The listing builds one solid part. Answer for the finished solid, in the listing's coordinates (mm). Face numbers are marked on the shaded views. A direction names the side the tool comes from. Give positions to 0.01 mm unless a question says otherwise; leave off trailing zeros. Write each loop counter-clockwise with the first axis right and the second up, starting at its lowest first coordinate (ties: lowest second). Pieces come first, ordered by that corner, then holes. Notation, with made-up numbers: (46.5, 62) - (102.5, 62) arc R17 cw to (102.5, 71) - close; hole circle Ø7 at (-27.5, 65.5). An arc over 180 degrees is marked (long way). Return JSON: item names as keys, results as strings.
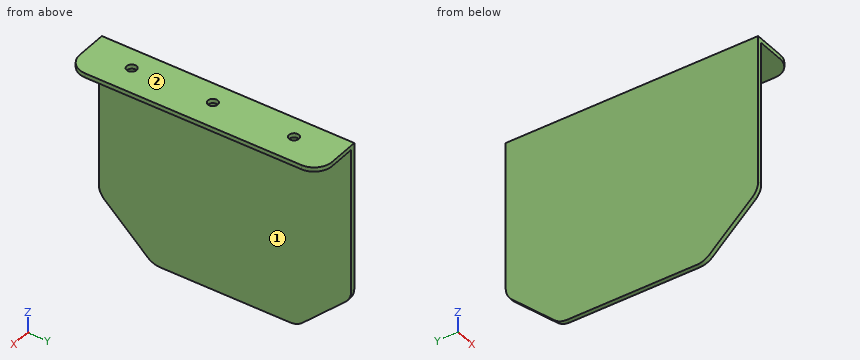
from build123d import *

# Parameters (mm, degrees)
SKETCH1_W           = 115
SKETCH1_H           = 140
BOSS_EXTRUDE1_DEPTH = 2.4
CUT_EXTRUDE1_DEPTH  = 3.4
FILLET1_R           = 10
SKETCH3_W           = 2.4
SKETCH3_H           = 140
BOSS_EXTRUDE2_DEPTH = 25
FILLET2_R           = 10
SKETCH4_R           = 2.75
CUT_EXTRUDE2_DEPTH  = 116


with BuildPart() as part:
    # Sketch1 → Boss-Extrude1 (new body)
    with BuildSketch(Plane(origin=(0, 0, 0), x_dir=(0, 0, -1), z_dir=(1, 0, 0))):
        with Locations((57.5, -70)):
            Rectangle(SKETCH1_W, SKETCH1_H)
    extrude(amount=BOSS_EXTRUDE1_DEPTH)

    # Sketch2 → Cut-Extrude1 (cut, through all)
    with BuildSketch(Plane(origin=(2.4, 0, 0), x_dir=(0, 0, -1), z_dir=(1, 0, 0))):
        Polygon((87, 0), (115, -30), (142.616199658, -32.505405645), (142.616199658, 14.875556406), align=None)
        Polygon((115, -110), (87, -140), (87, -152.661109726), (136.310004643, -152.661109726), align=None)
    extrude(amount=-CUT_EXTRUDE1_DEPTH, mode=Mode.SUBTRACT)

    # Fillet1
    fillet1_edges = [part.edges().sort_by_distance(p)[0] for p in [
        (1.2, 0, -87),
        (1.2, -30, -115),
        (1.2, -110, -115),
        (1.2, -140, -87),
    ]]
    fillet(fillet1_edges, radius=FILLET1_R)

    # Sketch3 → Boss-Extrude2 (add)
    with BuildSketch(Plane(origin=(2.4, 0, 0), x_dir=(0, 0, -1), z_dir=(1, 0, 0))):
        with Locations((1.2, -70)):
            Rectangle(SKETCH3_W, SKETCH3_H)
    extrude(amount=BOSS_EXTRUDE2_DEPTH)

    # Fillet2
    fillet2_edges = [part.edges().sort_by_distance(p)[0] for p in [
        (27.4, -140, -1.2),
        (27.4, 0, -1.2),
    ]]
    fillet(fillet2_edges, radius=FILLET2_R)

    # Sketch4 → Cut-Extrude2 (cut, through all)
    with BuildSketch(Plane.XY):
        with Locations((11.974983581, -70)):
            Circle(SKETCH4_R)
        with Locations((11.974983581, -25)):
            Circle(SKETCH4_R)
        with Locations((11.974983581, -115)):
            Circle(SKETCH4_R)
    extrude(amount=-CUT_EXTRUDE2_DEPTH, mode=Mode.SUBTRACT)


solid = part.part
Item 1: A cutting plane is placed at A-A on y = -115. Determine the outline of the cut face in (x, z), then the cut area to 3 significant figures.
Answer below:
{"outline": "(0, -110.33) - (2.4, -110.33) - (2.4, -2.4) - (9.22, -2.4) - (9.22, 0) - (0, 0) - close; (14.72, -2.4) - (27.4, -2.4) - (27.4, 0) - (14.72, 0) - close", "area": "312 mm²"}
Item 2: For the marked faces 1 and 2, determine the directions among +Z, -Z, +X, -X, +Y, -Y from which every point of the face is accessible in a straight line to the end or side of a thin tool.
Answer below:
{"face 1": "-Z, +X, +Y, -Y", "face 2": "+Z, +X, -X, +Y, -Y"}
Item 3: A cutting plane is placed at C-C on y = -93. Determine the outline of the cut face in (x, z), then the cut area to 3 significant figures.
Answer below:
{"outline": "(0, -115) - (2.4, -115) - (2.4, -2.4) - (27.4, -2.4) - (27.4, 0) - (0, 0) - close", "area": "336 mm²"}
Item 4: A cutting plane is placed at D-D on x = 4. Determine the outline of the cut face in (y, z).
Answer below:
{"outline": "(-140, -2.4) - (0, -2.4) - (0, 0) - (-140, 0) - close"}
Item 5: Consider L1, parallel to Z at x = 5.25, y = -30.5; L2, parallel to X at y = -68.5, z = -75.5; L3, parallel to Z at x = 2.25, y = -118.5. Determine where each line is inside the solid, lowest interval first.
Answer below:
{"L1": "z = -2.4 to 0", "L2": "x = 0 to 2.4", "L3": "z = -107.07 to 0"}
Item 6: A cutting plane is placed at B-B on x = 13. Determine the outline of the cut face in (y, z).
Answer below:
{"outline": "(-140, -2.4) - (-117.55, -2.4) - (-117.55, 0) - (-140, 0) - close; (-112.45, -2.4) - (-72.55, -2.4) - (-72.55, 0) - (-112.45, 0) - close; (-67.45, -2.4) - (-27.55, -2.4) - (-27.55, 0) - (-67.45, 0) - close; (-22.45, -2.4) - (0, -2.4) - (0, 0) - (-22.45, 0) - close"}
Item 7: Flat-ended cylindrical pins translate along their axes: P1, Ø12, axis at x = 4.5, y = -52.5, coming from the -Z side; P2, Ø2, axis at y = -84.5, z = -64, coming from the +X side; P3, Ø4.5, axis at x = 11.97, y = -70, coming from the +Z side. Find the tip coordinate at first contact, or state that the pin passes through.
Answer below:
{"P1": "stops at z = -115", "P2": "stops at x = 2.4", "P3": "passes through"}
